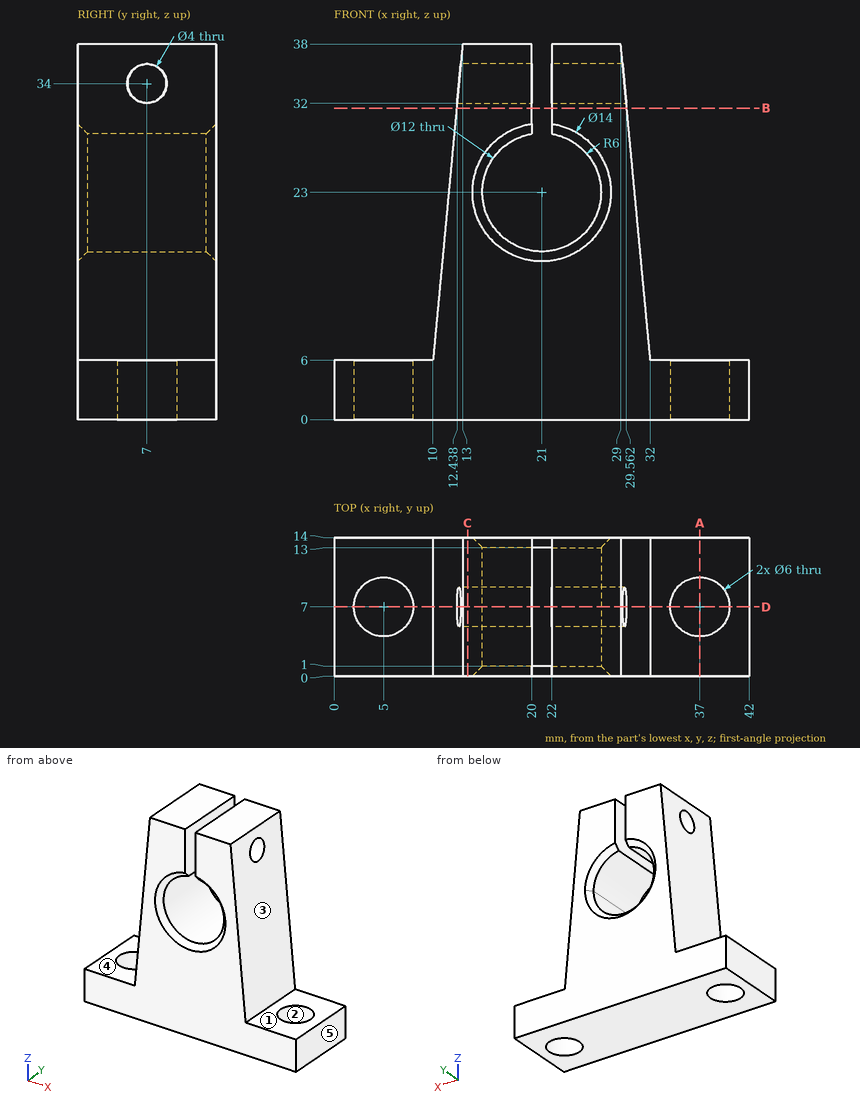
Answer from the drawing. Dimensions are ordinates in mm from the lowest x, y and z of the part. A direction names the side the tool comes from. Coordinates: 2 decimals unless noted, no trailing zeros. Loops run counter-clockwise (first coordinate to the right, second up) from the corner with the lowest first, then second, coordinate; pieces in that order, holes last. Notation, with made-up numbers: (-2.5, 12.5) - (33.5, 12.5) arc R12 cw to (33.5, 21.5) - close; hole circle Ø8 at (-16, 27.5). An arc over 180 degrees is marked (long way). Answer in a Markdown table with one row per item.
1. Find section C-C, the plane x = 13.5. Write down the section's boundary in (y, z).
Conclusion:
| item | result |
|---|---|
| outline | (0, 0) - (14, 0) - (14, 38) - (0, 38) - close; hole circle Ø4 at (7, 34) |
2. Given pin 1 (4.5 mm diameter, centred on y = 7, z = 34, fed in from +X); pin 2 (2.5 mm diameter, centred on y = 8, z = 35.5, fed in from +X); pin 3 (8 mm diameter, centred on x = 5.5, y = 9.5, fed in from +Z); pin 4 (10 mm diameter, centred on x = 8.5, z = 9.5, fed in from -Y), each flat-ended and moving along its own axis, determine where each tip first touches the part or whether it passes through.
Conclusion:
| item | result |
|---|---|
| pin 1 | stops at x = 29.59 |
| pin 2 | stops at x = 29.32 |
| pin 3 | stops at z = 6 |
| pin 4 | stops at y = 0 |
3. Find section A-A, the plane x = 37. Write down the section's boundary in (y, z), then the cut area to 3 significant figures.
Conclusion:
| item | result |
|---|---|
| outline | (0, 0) - (4, 0) - (4, 6) - (0, 6) - close; (10, 0) - (14, 0) - (14, 6) - (10, 6) - close |
| area | 48.0 mm² |
4. Find section B-B, the plane z = 31.5. Write down the section's boundary in (x, y).
Conclusion:
| item | result |
|---|---|
| outline | (12.39, 0) - (20, 0) - (20, 14) - (12.39, 14) - close; (22, 0) - (29.61, 0) - (29.61, 14) - (22, 14) - close |
5. Determine the mould class of the marked faces 1, 2 and 3 for opening direction X: +X half, -X half, draft (parallel to the pull), parting line (faces both ways), or undercut.
Conclusion:
| item | result |
|---|---|
| face 1 | draft |
| face 2 | undercut |
| face 3 | +X half |
6. Straight lines are drawn through the part: line 1 (X direction, y = 7, z = 4.7); line 2 (X direction, y = 5.5, z = 5.5); line 3 (Y direction, x = 37, z = 3.85). For each, find the intervals that lie inside material, in ascending order.
Conclusion:
| item | result |
|---|---|
| line 1 | x = 0 to 2, 8 to 34, 40 to 42 |
| line 2 | x = 0 to 2.4, 7.6 to 34.4, 39.6 to 42 |
| line 3 | y = 0 to 4, 10 to 14 |
7. Which of the six approach directions +Z, -Z, +X, -X, +Y, -Y give full straight-line access (tool end or side, diameter ignored) to the marked faces 4 and 5?
Conclusion:
| item | result |
|---|---|
| face 4 | +Z, -X, +Y, -Y |
| face 5 | +Z, -Z, +X, +Y, -Y |
8. Find section D-D, the plane y = 7. Write down the section's boundary in (x, z), then the cut area to 3 significant figures.
Conclusion:
| item | result |
|---|---|
| outline | (0, 0) - (2, 0) - (2, 6) - (0, 6) - close; (8, 0) - (34, 0) - (34, 6) - (32, 6) - (29.56, 32) - (22, 32) - (22, 28.92) arc R6 cw (long way) to (20, 28.92) - (20, 32) - (12.44, 32) - (10, 6) - (8, 6) - close; (12.81, 36) - (20, 36) - (20, 38) - (13, 38) - close; (22, 36) - (29.19, 36) - (29, 38) - (22, 38) - close; (40, 0) - (42, 0) - (42, 6) - (40, 6) - close |
| area | 598 mm² |
